from build123d import *

# Parameters (mm, degrees)
SZKIC1_W                    = 90
SZKIC1_H                    = 90
SZKIC1_R                    = 6
DODANIE_WYCI_GNI_CIE1_DEPTH = 12
SZKIC2_W                    = 120
SZKIC2_H                    = 120
SZKIC2_W_2                  = 90
SZKIC2_H_2                  = 90
DODANIE_WYCI_GNI_CIE3_DEPTH = 12


with BuildPart() as part:
    # Szkic1 → Dodanie-wyciągnięcie1 (new body)
    with BuildSketch(Plane.XY):
        with Locations((10.517420564, -9.685096154)):
            Rectangle(SZKIC1_W, SZKIC1_H)
        with Locations((-24.583084499, 25.41540891)):
            Circle(SZKIC1_R, mode=Mode.SUBTRACT)
        with Locations((-24.583084499, -44.785601217)):
            Circle(SZKIC1_R, mode=Mode.SUBTRACT)
        with Locations((45.617925627, -44.785601217)):
            Circle(SZKIC1_R, mode=Mode.SUBTRACT)
        with Locations((45.617925627, 25.41540891)):
            Circle(SZKIC1_R, mode=Mode.SUBTRACT)
    extrude(amount=DODANIE_WYCI_GNI_CIE1_DEPTH)

    # Szkic2 → Dodanie-wyciągnięcie3 (add)
    with BuildSketch(Plane.XY.offset(12)):
        with Locations((10.517420564, -9.685096154)):
            Rectangle(SZKIC2_W, SZKIC2_H)
        with Locations((10.517420564, -9.685096154)):
            Rectangle(SZKIC2_W_2, SZKIC2_H_2, mode=Mode.SUBTRACT)
    extrude(amount=-DODANIE_WYCI_GNI_CIE3_DEPTH)


solid = part.part
Can you work these out from the model? Positions are in its coordinate system, mm. Give positions to 0.01 mm unless a question says otherwise; leave off trailing zeros. Loops run counter-clockwise (first coordinate to the right, second up) from the corner with the lowest first, then second, coordinate; pieces in that order, holes last. Notation, with made-up numbers: (75.5, 62.5) -> (131.5, 62.5) arc R24 cw to (131.5, 97.5) -> close; hole circle Ø11 at (77, -9.75). An arc over 180 degrees is marked (long way). Write item = value, one per line.
1) Suppose I cut it at A-A on z = 4.25. Write out the boundary of the cut face in (x, y), then the cut area to 3 significant figures.
Check result:
outline = (-49.48, -69.69) -> (70.52, -69.69) -> (70.52, 50.31) -> (-49.48, 50.31) -> close; hole circle Ø12 at (-24.58, -44.79); hole circle Ø12 at (-24.58, 25.42); hole circle Ø12 at (45.62, -44.79); hole circle Ø12 at (45.62, 25.42)
area = 13,900 mm2
2) I need wall thicknesses on L1, parallel to Y at x = -27.5, z = 9; L2, parallel to Y at x = -22.5, z = 10.25; L3, parallel to X at y = -49.5, z = 10. Which ranges of each line are inside material? Lowest first, please. Write a range as from..to.
Check result:
L1 = -69.69..-50.03, -39.54..20.17, 30.66..50.31
L2 = -69.69..-50.41, -39.16..19.79, 31.04..50.31
L3 = -49.48..-28.29, -20.87..41.91, 49.33..70.52
3) Thinking about a two-plate mould opening in X: for faces 1 (the flat face through (70.517, -11, 6)), 2 (the flat face through (10, -9, 0)), 3 (the cylindrical face through (-21.8, -50.1, 5.9)), which applies, released by +X, released by -X, zero draft, split by the parting line, or undercut?
Check result:
face_1 = released by +X
face_2 = zero draft
face_3 = undercut
4) Will these pins go through, and if not, where does the flat tip stop? pin 1 (12 mm diameter, centred on x = 17.5, y = -40, fed in from -Z); pin 2 (9.5 mm diameter, centred on x = 45.62, y = 25.42, fed in from +Z).
Check result:
pin_1 = 0
pin_2 = through
